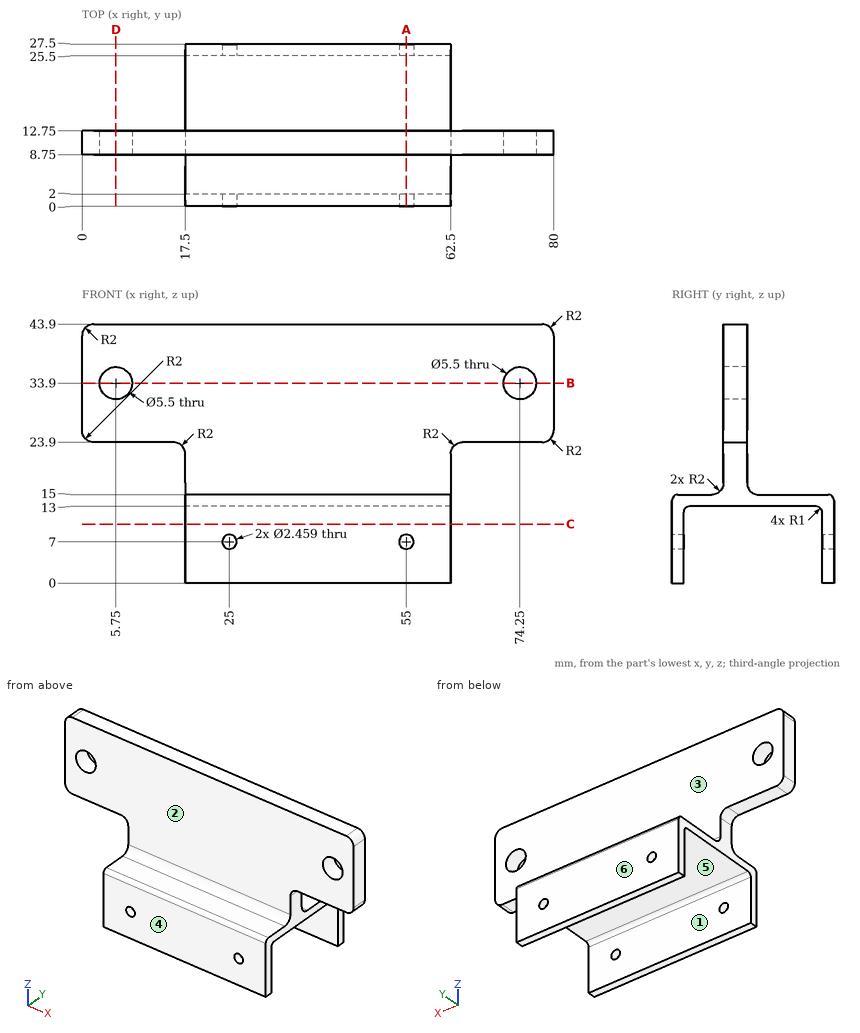
Job drawing, mm, ordinate dimensions from the low corner. One solid piece. A direction names the side the tool comes from. Coordinates: 2 decimals unless noted, no trailing zeros. Loops run counter-clockwise (first coordinate to the right, second up) from the corner with the lowest first, then second, coordinate; pieces in that order, holes last. Notation, with made-up numbers: (-32.5, 31) -> (8.5, 31) arc R25 cw to (8.5, 46) -> close; hole circle Ø9 at (63.25, 41). An arc over 180 degrees is marked (long way). One line per item, written item: value.
1. Slice it at B-B on z = 33.9. Write the cut outline in (x, y), and give its area (3 significant figures).
Answers:
outline: (0, 8.75) -> (3, 8.75) -> (3, 12.75) -> (0, 12.75) -> close; (8.5, 8.75) -> (71.5, 8.75) -> (71.5, 12.75) -> (8.5, 12.75) -> close; (77, 8.75) -> (80, 8.75) -> (80, 12.75) -> (77, 12.75) -> close
area: 276 mm^2
2. Slice it at A-A on x = 55. Write the cut outline in (y, z).
Answers:
outline: (0, 0) -> (2, 0) -> (2, 5.77) -> (0, 5.77) -> close; (0, 8.23) -> (2, 8.23) -> (2, 12) arc R1 cw to (3, 13) -> (24.5, 13) arc R1 cw to (25.5, 12) -> (25.5, 8.23) -> (27.5, 8.23) -> (27.5, 14) arc R1 ccw to (26.5, 15) -> (14.75, 15) arc R2 cw to (12.75, 17) -> (12.75, 43.9) -> (8.75, 43.9) -> (8.75, 17) arc R2 cw to (6.75, 15) -> (1, 15) arc R1 ccw to (0, 14) -> close; (25.5, 0) -> (27.5, 0) -> (27.5, 5.77) -> (25.5, 5.77) -> close
3. Slice it at D-D on x = 5.75. Write the cut outline in (y, z), and give its area (3 significant figures).
Answers:
outline: (8.75, 23.9) -> (12.75, 23.9) -> (12.75, 31.15) -> (8.75, 31.15) -> close; (8.75, 36.65) -> (12.75, 36.65) -> (12.75, 43.9) -> (8.75, 43.9) -> close
area: 58.0 mm^2
4. Slice it at C-C on z = 10. Write the cut outline in (x, y), and give its area (3 significant figures).
Answers:
outline: (17.5, 0) -> (62.5, 0) -> (62.5, 2) -> (17.5, 2) -> close; (17.5, 25.5) -> (62.5, 25.5) -> (62.5, 27.5) -> (17.5, 27.5) -> close
area: 180 mm^2
5. Drill centre lines: line 1 (X direction, y = 0.45, z = 7); line 2 (Y direction, x = 46.5, z = 5); line 3 (Z direction, x = 55, y = 1.2). Where is each one in solid material? Low to high. Write a range as [from, to].
Answers:
line 1: x = [17.5, 23.77], [26.23, 53.77], [56.23, 62.5]
line 2: y = [0, 2], [25.5, 27.5]
line 3: z = [0, 5.77], [8.23, 15]
6. Flat gauge pins, fed straight in: P1, Ø3, axis at x = 56.5, y = 11.5, coming from the -Z side; P2, Ø10, axis at y = 9.5, z = 11, coming from the -X side; P3, Ø13.5, axis at x = 26, z = 24.5, coming from the +Y side; P4, Ø2, axis at x = 55, z = 7, coming from the +Y side. Where does each tip first touch, or does it go through?
Answers:
P1: stops at z = 13
P2: stops at x = 17.5
P3: stops at y = 12.75
P4: passes through
7. Which spindle directions (+Z, -Z, +X, -X, +Y, -Y) get a long thin tool onto all of the face, cutting with end or side? Do the marked faces 1, 2 and 3. Say none if no direction does.
Answers:
face 1: -Z, +X, -X
face 2: +Z, +X, -X, -Y
face 3: +Z, +X, -X, +Y
8. Pull direction Y, two halves, no side cores. Call the marked faces 4, 5 and 6: pulls with the +Y half, pulls with the -Y half, needs draft (parallel to the pull), parting line crosses it, or undercut.
Answers:
face 4: pulls with the -Y half
face 5: undercut
face 6: pulls with the +Y half
